The listing builds one solid part. Answer for the finished solid, in the listing's coordinates (mm). A direction names the side the tool comes from. Give positions to 0.01 mm unless a question says otherwise; leave off trailing zeros. Loops run counter-clockwise (first coordinate to the right, second up) from the corner with the lowest first, then second, coordinate; pieces in that order, holes last. Notation, with made-up numbers: (-40, 82.5) - (-36, 82.5) arc R17 ccw to (-36, 108.5) - close; hole circle Ø2 at (-1.5, 7). An arc over 180 degrees is marked (long way). Answer in a Markdown table with one row per item. Add a question column.
Autodesk Inventor part; units mm, degrees
ref_plane "YZ Plane" through (0, 0, 0) normal (1, 0, 0) x (0, 1, 0)
ref_plane "XZ Plane" through (0, 0, 0) normal (0, 1, 0) x (-1, 0, 0)
ref_plane "XY Plane" through (0, 0, 0) normal (0, 0, 1) x (1, 0, 0)
sketch "Sketch3" plane through (0, 0, 0) normal (0, 0, 1) x (1, 0, 0)
  line L0 (0, 25.4) -> (0, -25.4)
  line L1 (0, 25.4) -> (19.05, 25.4)
  line L2 (19.05, 25.4) -> (19.05, 22.225)
  line L3 (19.05, 22.225) -> (3.048, 22.225)
  line L4 (3.048, 22.225) -> (3.048, -22.225)
  line L5 (3.048, -22.225) -> (19.05, -22.225)
  line L6 (19.05, -22.225) -> (19.05, -25.4)
  line L7 (19.05, -25.4) -> (0, -25.4)
  line L8 (0, 0) -> (3.048, 0) construction
  dimension "d7" = 50.8
  dimension "d10" = 19.05
  dimension "d33" = 3.175
  dimension "d34" = 16.002
extrude "Extrusion3" add sketch "Sketch3" along normal mid plane 660.4
fillet "Fillet1" radius 1.5875 4 edges at (19.05, 22.225, 0) (19.05, -22.225, 0) (3.048, -22.225, 0) (3.048, 22.225, 0)
sketch "Sketch6" plane through (0, -25.4, 330.2) normal (-1, 0, 0) x (0, 0, 1)
  line L0 (-496.189, 3.81) -> (-453.009, 3.81)
  line L1 (-453.009, 3.81) -> (-453.009, 46.99)
  line L2 (-453.009, 46.99) -> (-496.189, 46.99)
  line L3 (-496.189, 46.99) -> (-496.189, 3.81)
  line L4 (-496.189, 3.81) -> (-453.009, 46.99) construction
  line L5 (-453.009, 3.81) -> (-496.189, 46.99) construction
  line L6 (-207.391, 3.81) -> (-164.211, 3.81)
  line L7 (-164.211, 3.81) -> (-164.211, 46.99)
  line L8 (-164.211, 46.99) -> (-207.391, 46.99)
  line L9 (-207.391, 46.99) -> (-207.391, 3.81)
  line L10 (-207.391, 3.81) -> (-164.211, 46.99) construction
  line L11 (-164.211, 3.81) -> (-207.391, 46.99) construction
  point P0 (-330.2, 25.4)
  point P1 (-474.599, 25.4)
  point P2 (-185.801, 25.4)
  point P3 (-474.599, 25.4)
  point P4 (-185.801, 25.4)
  dimension "d35" = 288.798
  dimension "d36" = 144.399
  dimension "d37" = 43.18
extrude "Extrusion4" cut sketch "Sketch6" against normal through all
sketch "Sketch7" plane through (3.048, -20.6375, 330.2) normal (1, 0, 0) x (0, 0, -1)
  circle A0 centre (227.075, 4.7625) radius 2.4194
  circle A1 centre (227.075, 36.5125) radius 2.4194
  circle A2 centre (144.525, 4.7625) radius 2.4194
  circle A3 centre (144.525, 36.5125) radius 2.4194
  circle A4 centre (515.875, 4.7625) radius 2.4194
  circle A5 centre (515.875, 36.5125) radius 2.4194
  circle A6 centre (433.325, 4.7625) radius 2.4194
  circle A7 centre (433.325, 36.5125) radius 2.4194
  point P0 (330.2, 20.6375)
hole "Hole3" at (3.048, -15.875, -185.675) at (3.048, 15.875, -185.675) at (3.048, -15.875, -103.125) at (3.048, 15.875, -103.125) at (3.048, -15.875, 103.125) at (3.048, 15.875, 103.125) at (3.048, -15.875, 185.675) at (3.048, 15.875, 185.675) direction (-1, 0, 0) diameter 6.7564 end through all
equation "\"d11\" = Length"
equation "\"Length\" = 660.4"
properties part number "NASA-20-FR-SP-01" material "Aluminum 6061"
(1) Find the intervals of material crossed by line 1 along Y through (x, z) = (10.25, 196.5) (3 decimals); line 2 along Y through (x, z) = (18, 228); line 3 along X through (y, z) = (5.5, 89.5), in increasing order. Write a range as [from, to].
(2) A cutting plane is placed at B-B on x = 10.75. Determine the outline of the cut face in (y, z) (3 decimals), plus the area to 3 significant figures.
(3) A tool of negligible diameter and unlimited length cuts with its end or side. For faces 5 (the face through (0, 0, -5)), 6 (the face through (3.048, 0, -2)), from which of +Z, -Z, +X, -X, +Y, -Y can it reach the whole face along a straight path? Write none if from no direction.
(4) A cutting plane is placed at A-A on y = -3. Determine the outline of the cut face in (x, z), plus the area to 3 significant figures.
(5) Given pin 1 Ø4 at (x, y) = (7, -19.5) entering from +Z; pin 2 Ø8 at (y, z) = (15.875, -185.675) entering from +X; pin 3 Ø12 at (y, z) = (17.5, 239) entering from +X; pin 4 Ø10 at (x, y) = (15, 19.5) entering from +Z, each flat-ended and moving along its own axis, determine where each tip first touches the part or whether it passes through.
(6) The mould has two halves that part along Y. Classify faces 1 (the face through (10, -25.4, -5)), 2 (the face through (3.048, 0, -249)), 3 (the face through (9, 25.4, -5)), 4 (the face through (2, 2, 330.2)): pulls with the +Y half, pulls with the -Y half, needs draft (parallel to the pull), parting line crosses it, or undercut.
Evaluation:
| question | item | result |
|---|---|---|
| 1 | line 1 | y = [-25.4, -22.225], [22.225, 25.4] |
| 1 | line 2 | y = [-25.4, -22.32], [22.32, 25.4] |
| 1 | line 3 | x = [0, 3.05] |
| 2 | outline | (-25.4, -330.2) - (-22.225, -330.2) - (-22.225, 330.2) - (-25.4, 330.2) - close; (22.225, -330.2) - (25.4, -330.2) - (25.4, 330.2) - (22.225, 330.2) - close |
| 2 | area | 4,190 mm² |
| 3 | face 5 | +Z, -Z, -X, +Y, -Y |
| 3 | face 6 | +Z, -Z, +X |
| 4 | outline | (0, -330.2) - (3.05, -330.2) - (3.05, -165.99) - (0, -165.99) - close; (0, -122.81) - (3.05, -122.81) - (3.05, 122.81) - (0, 122.81) - close; (0, 165.99) - (3.05, 165.99) - (3.05, 330.2) - (0, 330.2) - close |
| 4 | area | 1,750 mm² |
| 5 | pin 1 | passes through |
| 5 | pin 2 | stops at x = 3.05 |
| 5 | pin 3 | stops at x = 19.02 |
| 5 | pin 4 | stops at z = 330.2 |
| 6 | face 1 | pulls with the -Y half |
| 6 | face 2 | undercut |
| 6 | face 3 | pulls with the +Y half |
| 6 | face 4 | needs draft |
